from build123d import *

# Parameters (mm, degrees)
F1_DEPTH = 3.048
F2_W     = 40
F2_H     = 9
F3_DEPTH = 2
F4_W     = 40
F4_H     = 9
F5_DEPTH = 2
F7_D     = 2.5


with BuildPart() as f1:
    # F0 (on Front) → F1 (new body, symmetric)
    with BuildSketch(Plane.XZ):
        Polygon((-12.75, 0), (-20, 0), (-20, -6), (20, -6), (20, 0), (12.75, 0), (12.75, 3), (-12.75, 3), align=None)
    extrude(amount=F1_DEPTH, both=True)

    # F2 (on face) → F3 (join)
    with BuildSketch(Plane.XZ.offset(3.048)):
        with Locations((0, -1.5)):
            Rectangle(F2_W, F2_H)
    extrude(amount=F3_DEPTH)

    # F4 (on face) → F5 (join)
    with BuildSketch(Plane(origin=(0, 3.048, 0), x_dir=(-1, 0, 0), z_dir=(0, 1, 0))):
        with Locations((0, -1.5)):
            Rectangle(F4_W, F4_H)
    extrude(amount=F5_DEPTH)

    # F7 (through all)
    with Locations(Plane.XY):
        with Locations((-15, 0), (15, 0)):
            Hole(F7_D / 2)


solid = f1.part
Could you check a few things on this model? Use its own coordinates, in mm. A direction names the side the tool comes from. Give positions to 0.01 mm unless a question says otherwise; leave off trailing zeros. Write each loop counter-clockwise with the first axis right and the second up, starting at its lowest first coordinate (ties: lowest second). Pieces come first, ordered by that corner, then holes. Notation, with made-up numbers: (65.25, 76.5) - (87.25, 76.5) arc R36 cw to (87.25, 115.5) - close; hole circle Ø4 at (15.5, 42.25). An arc over 180 degrees is marked (long way). Use CSV: the item, a comma, the result in double quotes. Start each with the question number.
Item 1: If we mould it in two halves opening along Y, with no side actions, what happens to faces 4 (the face through (-17, 0, 0)), 5 (the face through (0, -5.048, -1)), 6 (the face through (20, 0, -3))? For each: pulls with the +Y half, pulls with the -Y half, needs draft (parallel to the pull), parting line crosses it, or undercut.
Item 2: I'm going to push flat-ended pins straight in: pin 1 (3 mm diameter, centred on x = -17.5, y = 1, fed in from +Z); pin 2 (1.5 mm diameter, centred on x = -15, y = 0, fed in from +Z); pin 3 (2.5 mm diameter, centred on y = -0.5, z = 2, fed in from +X); pin 4 (2.5 mm diameter, centred on y = 1, z = 1.5, fed in from -X). Where does each tip first touch, or does it pass through?
Item 3: I want a section at C-C, the plane z = -2. Please give me the cut outline in (x, y).
Item 4: I want a section at D-D, the plane z = 0.75. Please give me the cut outline in (x, y).
Item 5: For faces 1 (the face through (-16, 3.048, 2)), 2 (the face through (16, 3.048, 2)), 3 (the face through (-20, 0, -3)), which set-ups out of +Z, -Z, +X, -X, +Y, -Y let a thin tool reach every point of the face, with its end or its side?
Item 6: I want a section at A-A, the plane y = 0. Please give me the cut outline in (x, z), then the cut area to 4 significant figures.
Item 7: I want a section at B-B, the plane x = -15. Please give me the cut outline in (y, z).
Item 8: If I drill on line 1 along Y through (x, z) = (15, -4.35); line 2 along X through (y, z) = (1, -3.5); line 3 along Z through (x, y) = (-16, -1), over which ranges is the centre line in solid material (lowest first)?
Findings:
1,face 4,"undercut"
1,face 5,"pulls with the -Y half"
1,face 6,"needs draft"
2,pin 1,"stops at z = 0"
2,pin 2,"passes through"
2,pin 3,"stops at x = 12.75"
2,pin 4,"stops at x = -12.75"
3,outline,"(-20, -5.05) - (20, -5.05) - (20, 5.05) - (-20, 5.05) - close; hole circle Ø2.5 at (-15, 0); hole circle Ø2.5 at (15, 0)"
4,outline,"(-20, -5.05) - (20, -5.05) - (20, -3.05) - (12.75, -3.05) - (12.75, 3.05) - (20, 3.05) - (20, 5.05) - (-20, 5.05) - (-20, 3.05) - (-12.75, 3.05) - (-12.75, -3.05) - (-20, -3.05) - close"
5,face 1,"+Z, -X"
5,face 2,"+Z, +X"
5,face 3,"+Z, -Z, -X, +Y, -Y"
6,outline,"(-20, -6) - (-16.25, -6) - (-16.25, 0) - (-20, 0) - close; (-13.75, -6) - (13.75, -6) - (13.75, 0) - (12.75, 0) - (12.75, 3) - (-12.75, 3) - (-12.75, 0) - (-13.75, 0) - close; (16.25, -6) - (20, -6) - (20, 0) - (16.25, 0) - close"
6,area,"286.5 mm2"
7,outline,"(-5.05, -6) - (-1.25, -6) - (-1.25, 0) - (-3.05, 0) - (-3.05, 3) - (-5.05, 3) - close; (1.25, -6) - (5.05, -6) - (5.05, 3) - (3.05, 3) - (3.05, 0) - (1.25, 0) - close"
8,line 1,"y = -5.05 to -1.25, 1.25 to 5.05"
8,line 2,"x = -20 to -15.75, -14.25 to 14.25, 15.75 to 20"
8,line 3,"z = -6 to 0"
